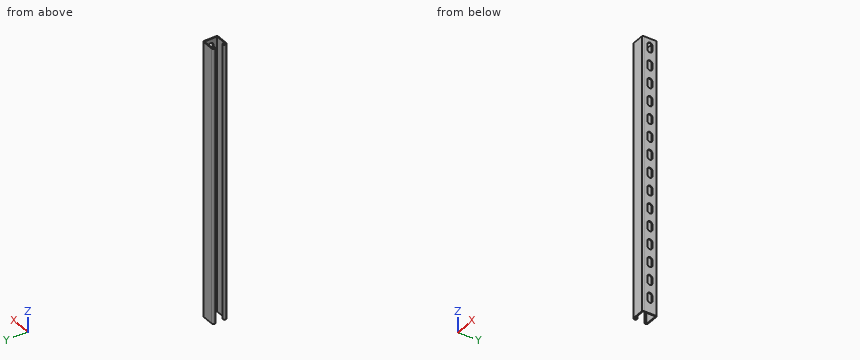
from build123d import *

# Parameters (mm, degrees)
BOSS_EXTRUDE1_DEPTH = 781.05
CUT_EXTRUDE1_DEPTH  = 2.794
LPATTERN1_COUNT     = 15
LPATTERN1_PITCH     = 50.8


with BuildPart() as part:
    # Sketch1 → Boss-Extrude1 (new body)
    with BuildSketch(Plane.XY):
        with BuildLine():
            Line((-36.22675, 20.6375), (-3.46075, 20.6375))
            ThreePointArc((-3.46075, 20.6375), (-1.013630207, 19.623869793), (0, 17.17675))
            Line((0, 17.17675), (0, -17.17675))
            ThreePointArc((0, -17.17675), (-1.013630207, -19.623869793), (-3.46075, -20.6375))
            Line((-3.46075, -20.6375), (-36.22675, -20.6375))
            ThreePointArc((-36.22675, -20.6375), (-39.796401808, -19.158901808), (-41.275, -15.58925))
            Line((-41.275, -15.58925), (-41.275, -14.57325))
            ThreePointArc((-41.275, -14.57325), (-40.261369793, -12.126130207), (-37.81425, -11.1125))
            Line((-37.81425, -11.1125), (-35.5346, -11.1125))
            ThreePointArc((-35.5346, -11.1125), (-34.1376, -12.5095), (-35.5346, -13.9065))
            Line((-35.5346, -13.9065), (-37.81425, -13.9065))
            ThreePointArc((-37.81425, -13.9065), (-38.285713446, -14.101786554), (-38.481, -14.57325))
            Line((-38.481, -14.57325), (-38.481, -15.58925))
            ThreePointArc((-38.481, -15.58925), (-37.820745461, -17.183245461), (-36.22675, -17.8435))
            Line((-36.22675, -17.8435), (-3.46075, -17.8435))
            ThreePointArc((-3.46075, -17.8435), (-2.989286554, -17.648213446), (-2.794, -17.17675))
            Line((-2.794, -17.17675), (-2.794, 17.17675))
            ThreePointArc((-2.794, 17.17675), (-2.989286554, 17.648213446), (-3.46075, 17.8435))
            Line((-3.46075, 17.8435), (-36.22675, 17.8435))
            ThreePointArc((-36.22675, 17.8435), (-37.820745461, 17.183245461), (-38.481, 15.58925))
            Line((-38.481, 15.58925), (-38.481, 14.57325))
            ThreePointArc((-38.481, 14.57325), (-38.285713446, 14.101786554), (-37.81425, 13.9065))
            Line((-37.81425, 13.9065), (-35.5346, 13.9065))
            ThreePointArc((-35.5346, 13.9065), (-34.1376, 12.5095), (-35.5346, 11.1125))
            Line((-35.5346, 11.1125), (-37.81425, 11.1125))
            ThreePointArc((-37.81425, 11.1125), (-40.261369793, 12.126130207), (-41.275, 14.57325))
            Line((-41.275, 14.57325), (-41.275, 15.58925))
            ThreePointArc((-41.275, 15.58925), (-39.796401808, 19.158901808), (-36.22675, 20.6375))
        make_face()
    extrude(amount=-BOSS_EXTRUDE1_DEPTH)

    # Sketch2 → Cut-Extrude1 (cut)
    with BuildSketch(Plane(origin=(0, 0, 0), x_dir=(0, 0, -1), z_dir=(1, 0, 0))):
        with BuildLine():
            Line((18.25625, 7.14375), (32.54375, 7.14375))
            ThreePointArc((32.54375, 7.14375), (39.6875, 0), (32.54375, -7.14375))
            Line((32.54375, -7.14375), (18.25625, -7.14375))
            ThreePointArc((18.25625, -7.14375), (11.1125, 0), (18.25625, 7.14375))
        make_face()
    cut_extrude1 = extrude(amount=-CUT_EXTRUDE1_DEPTH, mode=Mode.SUBTRACT)

    # LPattern1: Cut-Extrude1 ×15
    with Locations(*[(0, 0, -i * LPATTERN1_PITCH) for i in range(1, LPATTERN1_COUNT)]):
        add(cut_extrude1, mode=Mode.SUBTRACT)


solid = part.part
For this review, take the finished solid that the model builds, in its own axes (mm). Round coordinates to 2 decimals unless told otherwise and drop trailing zeros. Loops run counter-clockwise (first coordinate to the right, second up) from the corner with the lowest first, then second, coordinate; pieces in that order, holes last. Notation, with made-up numbers: (62.25, 85.25) - (72.25, 85.25) arc R15 cw to (72.25, 104.25) - close; hole circle Ø4 at (-8.75, -25). An arc over 180 degrees is marked (long way). Put each result on its own line as item: value. Start each with the question number.
1. Consider section A-A on x = -17.5. State the section outline as (y, z) points.
2. Insertion check: P1, Ø1.4, axis at x = -2, z = -380.5, coming from the -Y side; P2, Ø3, axis at x = -1.5, z = -483, coming from the +Y side; P3, Ø1.4, axis at x = -1, z = -737, coming from the +Y side. Each pin has a flat end and moves straight along its axis. Give the tip position at first contact, or say it passes through.
3. For probe 1 along X at (y, z) = (-15.5, -477) (3 decimals); probe 2 along Y at (x, z) = (-20, -671.5); probe 3 along X at (y, z) = (16, -708.5), list the stretches that pass through material, from the lowest coordinate up. Write a range as [from, to].
4. Consider section B-B on y = 0. State how many separate pieces and enclosed holes the cut face has, plus the area to 3 significant figures.
Result sheet:
1. outline: (-20.64, -781.05) - (-17.84, -781.05) - (-17.84, 0) - (-20.64, 0) - close; (17.84, -781.05) - (20.64, -781.05) - (20.64, 0) - (17.84, 0) - close
2. P1: y = -20.55
2. P2: y = 20.61
2. P3: y = 20.16
3. probe 1: [-41.275, -38.481], [-2.794, 0]
3. probe 2: [-20.64, -17.84], [17.84, 20.64]
3. probe 3: [-41.26, -38.44], [-2.79, 0]
4. separate pieces: 16
4. enclosed holes: 0
4. area: 985 mm^2
